Input: part model. Units: mm. Frame: model coordinates. Round coordinates to 2 decimals unless told otherwise and drop trailing zeros. Loops run counter-clockwise (first coordinate to the right, second up) from the corner with the lowest first, then second, coordinate; pieces in that order, holes last.
(1) First-contact query: pin 1 Ø1.2 at (x, z) = (-34, 11.5) entering from +Y; pin 2 Ø2 at (y, z) = (102, 12.5) entering from -X; pin 3 Ø1.2 at (y, z) = (-103, 13) entering from +X. Flat tips, straight axial feed; report the tip coordinate or a pass-through.
(2) Line query: line 1 (Y direction, x = -125, z = 11.85); line 2 (Y direction, x = -35.5, z = 11). Output: solid intervals per line, ascending.
(3) Cut plane A-A, the plane z = 12.55. Output: boundary loops of the cut face in (x, y), and give its area (3 significant figures).
(4) Cut plane B-B, the plane x = 70. Output: boundary loops of the cut face in (y, z).
from build123d import *

# Parameters (mm, degrees)
SKETCH1_R               = 3
SKETCH1_W               = 33
SKETCH1_H               = 80
BOSS_EXTRUDE1_DEPTH     = 14
SKETCH4_R               = 2
CUT_EXTRUDE2_DEPTH      = 10
SKETCH5_R               = 2
CUT_EXTRUDE3_DEPTH      = 10
SKETCH6_R               = 3
BOSS_EXTRUDE2_DEPTH     = 4
BOSS_EXTRUDE2_2_DEPTH   = 4
SKETCH7_R               = 6.85
SKETCH7_R_2             = 1.5
CUT_EXTRUDE4_DEPTH      = 10
ESQUISSE2_W             = 270
ESQUISSE2_H             = 10
ENL_V_MAT_EXTRU_1_DEPTH = 260
ESQUISSE3_W             = 4
ESQUISSE3_H             = 176.46718548
BOSS_EXTRU_3_DEPTH      = 265


with BuildPart() as part:
    # Sketch1 → Boss-Extrude1 (new body)
    with BuildSketch(Plane.XY):
        Polygon((-135, -20.635083269), (-135, -50), (135, -50), (135, -20.635083269), (135, 40), (135, 50), (-135, 50), (-135, 40), align=None)
        with Locations((-85, -43)):
            Circle(SKETCH1_R, mode=Mode.SUBTRACT)
        with Locations((-80, 43)):
            Circle(SKETCH1_R, mode=Mode.SUBTRACT)
        with Locations(Location((80, 43, 0), (0, 0, 180))):
            Circle(SKETCH1_R, mode=Mode.SUBTRACT)
        with Locations(Location((85, -43, 0), (0, 0, 180))):
            Circle(SKETCH1_R, mode=Mode.SUBTRACT)
        with Locations((-110.5, 0)):
            Rectangle(SKETCH1_W, SKETCH1_H, mode=Mode.SUBTRACT)
        Polygon((-61, -30), (-35, -30), (-35, -20), (-4, -20), (-4, 20), (-35, 20), (-35, 30), (-61, 30), align=None, mode=Mode.SUBTRACT)
        Polygon((35, 20), (35, 30), (61, 30), (61, -30), (35, -30), (35, -20), (4, -20), (4, 20), align=None, mode=Mode.SUBTRACT)
        with Locations((110.5, 5)):
            Rectangle(SKETCH1_W, SKETCH1_H, mode=Mode.SUBTRACT)
    extrude(amount=BOSS_EXTRUDE1_DEPTH)

    # Sketch4 → Cut-Extrude2 (cut)
    with BuildSketch(Plane(origin=(0, 0, 0), x_dir=(-1, 0, 0), z_dir=(0, 0, -1))):
        with Locations((-131.5, 5)):
            Circle(SKETCH4_R)
    cut_extrude2 = extrude(amount=-CUT_EXTRUDE2_DEPTH, mode=Mode.SUBTRACT)

    # Sketch5 → Cut-Extrude3 (cut)
    with BuildSketch(Plane(origin=(0, 0, 0), x_dir=(-1, 0, 0), z_dir=(0, 0, -1))):
        with Locations((-69, 5)):
            Circle(SKETCH5_R)
    cut_extrude3 = extrude(amount=-CUT_EXTRUDE3_DEPTH, mode=Mode.SUBTRACT)

    # Mirror1: Cut-Extrude2, Cut-Extrude3 across plane
    add(cut_extrude2.mirror(Plane.ZY), mode=Mode.SUBTRACT)
    add(cut_extrude3.mirror(Plane.ZY), mode=Mode.SUBTRACT)


with BuildPart() as body_2:
    # Sketch6 → Boss-Extrude2 (new body)
    with BuildSketch(Plane.XY.offset(14)):
        with BuildLine():
            Line((75, 110), (125, 110))
            ThreePointArc((125, 110), (132.071067812, 107.071067812), (135, 100))
            Line((135, 100), (135, 50))
            Line((135, 50), (-135, 50))
            Line((-135, 50), (-135, 100))
            ThreePointArc((-135, 100), (-132.071067812, 107.071067812), (-125, 110))
            Line((-125, 110), (-75, 110))
            Line((-75, 110), (-75, 95))
            Line((-75, 95), (75, 95))
            Line((75, 95), (75, 110))
        make_face()
        with Locations((-125, 95)):
            Circle(SKETCH6_R, mode=Mode.SUBTRACT)
        with Locations((125, 95)):
            Circle(SKETCH6_R, mode=Mode.SUBTRACT)
    extrude(amount=-BOSS_EXTRUDE2_DEPTH)

    # Combine1: union part
    add(part.part)


with BuildPart() as body_3:
    # Sketch6 → Boss-Extrude2 2 (new body)
    with BuildSketch(Plane.XY.offset(14)):
        with BuildLine():
            Line((75, -110), (75, -95))
            Line((75, -95), (-75, -95))
            Line((-75, -95), (-75, -110))
            Line((-75, -110), (-125, -110))
            ThreePointArc((-125, -110), (-132.071067812, -107.071067812), (-135, -100))
            Line((-135, -100), (-135, -50))
            Line((-135, -50), (135, -50))
            Line((135, -50), (135, -100))
            ThreePointArc((135, -100), (132.071067812, -107.071067812), (125, -110))
            Line((125, -110), (75, -110))
        make_face()
        with Locations(Location((125, -95, 0), (0, 0, 180))):
            Circle(SKETCH6_R, mode=Mode.SUBTRACT)
        with Locations(Location((-125, -95, 0), (0, 0, 180))):
            Circle(SKETCH6_R, mode=Mode.SUBTRACT)
    extrude(amount=-BOSS_EXTRUDE2_2_DEPTH)


with BuildPart() as body_2_1:
    add(body_2.part)

    # Combine2: union body 3
    add(body_3.part)

    # Sketch7 → Cut-Extrude4 (cut)
    with BuildSketch(Plane.XY.offset(14)):
        with Locations((0, 70)):
            Circle(SKETCH7_R)
        with Locations((-11.25, 76.495190528)):
            Circle(SKETCH7_R_2)
        with Locations((0, 57.009618943)):
            Circle(SKETCH7_R_2)
        with Locations((0, -70)):
            Circle(SKETCH7_R)
        with Locations((0, -57.009618943)):
            Circle(SKETCH7_R_2)
        with Locations(Location((11.25, 76.495190528, 0), (0, 0, 180))):
            Circle(SKETCH7_R_2)
        with Locations((-11.25, -76.495190528)):
            Circle(SKETCH7_R_2)
        with Locations((11.25, -76.495190528)):
            Circle(SKETCH7_R_2)
    extrude(amount=-CUT_EXTRUDE4_DEPTH, mode=Mode.SUBTRACT)

    # Esquisse2 → Enlèv. mat.-Extru.1 (cut)
    with BuildSketch(Plane.XZ.offset(50)):
        with Locations((0, 5)):
            Rectangle(ESQUISSE2_W, ESQUISSE2_H)
    extrude(amount=-ENL_V_MAT_EXTRU_1_DEPTH, mode=Mode.SUBTRACT)

    # Esquisse3 → Boss.-Extru.3 (add)
    with BuildSketch(Plane(origin=(135, 0, 0), x_dir=(0, 0, -1), z_dir=(1, 0, 0))):
        with Locations((-12, 0.244857916)):
            Rectangle(ESQUISSE3_W, ESQUISSE3_H)
    extrude(amount=-BOSS_EXTRU_3_DEPTH)


solid = body_2_1.part
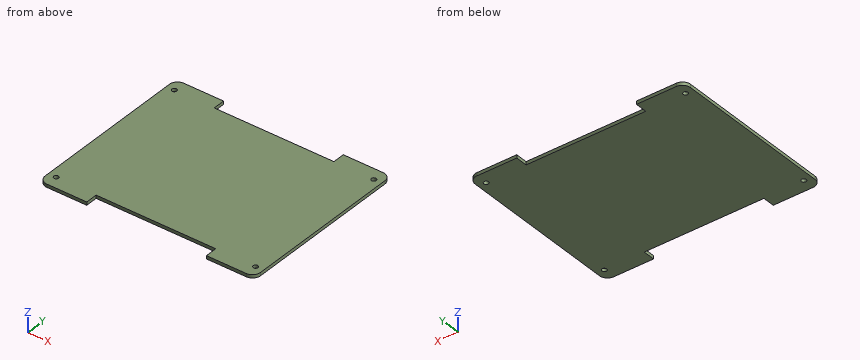
Reported:
1. pin 1: stops at y = 95
1. pin 2: stops at x = -134.95
1. pin 3: stops at x = 134.71
2. line 1: y = -110 to -98, -92 to 92, 98 to 110
2. line 2: y = -95 to 95
3. outline: (-135, -100) arc R10 ccw to (-125, -110) - (-75, -110) - (-75, -95) - (75, -95) - (75, -110) - (125, -110) arc R10 ccw to (135, -100) - (135, 100) arc R10 ccw to (125, 110) - (75, 110) - (75, 95) - (-75, 95) - (-75, 110) - (-125, 110) arc R10 ccw to (-135, 100) - close; hole circle Ø6 at (-125, -95); hole circle Ø6 at (-125, 95); hole circle Ø6 at (125, -95); hole circle Ø6 at (125, 95)
3. area: 54,700 mm2
4. outline: (-95, 10) - (95, 10) - (95, 14) - (-95, 14) - close
